```python
from build123d import *

# Parameters (mm, degrees)
F0_W     = 5.2
F0_H     = 226.71
F1_DEPTH = 2
F3_DEPTH = 4.5
F4_W     = 1.2
F4_H     = 2.1
F5_DEPTH = 25
F6_W     = 185.5
F6_H     = 227.71
F6_W_2   = 2.7
F7_DEPTH = 1
F8_W     = 2
F8_H     = 226.71
F9_DEPTH = 1
F10_SIZE = 1


with BuildPart() as f1:
    # F0 (on Top) → F1 (new body)
    with BuildSketch(Plane.XY):
        with Locations((2.6, 113.355)):
            Rectangle(F0_W, F0_H)
        with Locations((63.6, 113.355)):
            Rectangle(F0_W, F0_H)
        with Locations((124.6, 113.355)):
            Rectangle(F0_W, F0_H)
    extrude(amount=F1_DEPTH)

    # F2 (on face) → F3 (join)
    with BuildSketch(Plane.XY.offset(2)):
        Polygon((0, 226.71), (0, 0), (2, 0), (2, 224.71), (3.2, 224.71), (3.2, 0), (5.2, 0), (5.2, 226.71), align=None)
        Polygon((61, 226.71), (61, 0), (63, 0), (63, 224.71), (64.2, 224.71), (64.2, 0), (66.2, 0), (66.2, 226.71), align=None)
        Polygon((122, 226.71), (122, 0), (124, 0), (124, 224.71), (125.2, 224.71), (125.2, 0), (127.2, 0), (127.2, 226.71), align=None)
    extrude(amount=F3_DEPTH)

    # F4 (on face) → F5 (cut)
    with BuildSketch(Plane.XY.offset(2)):
        with Locations((2.6, 2.95)):
            Rectangle(F4_W, F4_H)
        with Locations((63.6, 2.95)):
            Rectangle(F4_W, F4_H)
        with Locations((124.6, 2.95)):
            Rectangle(F4_W, F4_H)
    extrude(amount=-F5_DEPTH, mode=Mode.SUBTRACT)

    # F6 (on Top) → F7 (join)
    with BuildSketch(Plane.XY):
        with Locations((34.45, 113.855)):
            Rectangle(F6_W, F6_H)
        with Locations((128.55, 113.855)):
            Rectangle(F6_W_2, F6_H)
    extrude(amount=-F7_DEPTH)

    # F8 (on face) → F9 (join)
    with BuildSketch(Plane.XY):
        with Locations((-53.8, 113.355)):
            Rectangle(F8_W, F8_H)
    extrude(amount=F9_DEPTH)

    # F10
    f10_edges = [f1.edges().sort_by_distance(p)[0] for p in [
        (2.6, 0, 2),
        (63.6, 0, 2),
        (124.6, 0, 2),
    ]]
    chamfer(f10_edges, length=F10_SIZE)


solid = f1.part
```
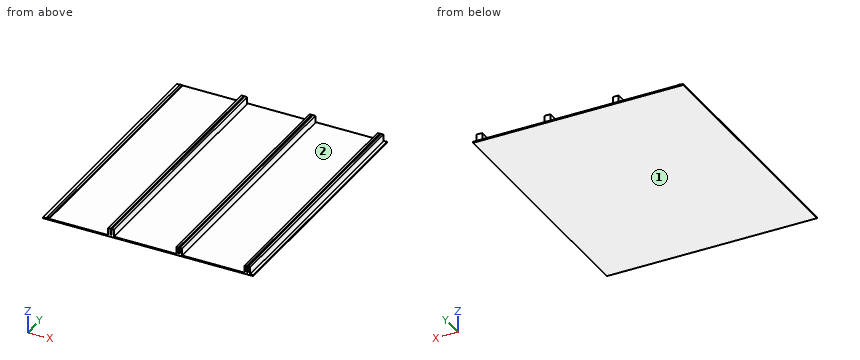
Here's how the part is built. I have some questions about the finished solid (model axes, mm). Face numbers are marked on the shaded views. Give positions to 0.01 mm unless a question says otherwise; leave off trailing zeros. Loops run counter-clockwise (first coordinate to the right, second up) from the corner with the lowest first, then second, coordinate; pieces in that order, holes last. Notation, with made-up numbers: M 67.25,67 L 114.25,67 A20 cw 114.25,102 Z; hole C -37,36 d2. An arc over 180 degrees is marked long. Put each result on its own line as item: value. Start each with the question number.
(1) I want a section at A-A on z = 4.25. Please give me the cut outline in (x, y).
(2) Will these pins go through, and if not, where does the flat tip stop? pin 1 Ø0.6 at (x, y) = (2.5, 133) entering from +Z; pin 2 Ø2 at (y, z) = (98, 1.5) entering from -X; pin 3 Ø2 at (y, z) = (98.5, 2) entering from +X; pin 4 Ø4 at (x, z) = (57.5, 3) entering from -Y.
(3) I want a section at C-C on x = 95. Please give me the cut outline in (y, z).
(4) If we mould it in two halves opening along X, with no side actions, what happens to the marked faces 1 and 2? For each: +X half, -X half, draft (parallel to the pull), parting line (faces both ways), or undercut.
(5) I need wall thicknesses on line 1 along X through (y, z) = (148, 3); line 2 along X through (y, z) = (114, 0.5); line 3 along X through (y, z) = (82, 1.5). Which ranges of each line are inside material? Lowest first, please. Write a range as [from, to].
Answer block:
1. outline: M 0,0 L 2,0 L 2,224.71 L 3.2,224.71 L 3.2,0 L 5.2,0 L 5.2,226.71 L 0,226.71 Z; M 61,0 L 63,0 L 63,224.71 L 64.2,224.71 L 64.2,0 L 66.2,0 L 66.2,226.71 L 61,226.71 Z; M 122,0 L 124,0 L 124,224.71 L 125.2,224.71 L 125.2,0 L 127.2,0 L 127.2,226.71 L 122,226.71 Z
2. pin 1: z = 2
2. pin 2: x = -54.8
2. pin 3: x = 127.2
2. pin 4: through
3. outline: M 0,-1 L 227.71,-1 L 227.71,0 L 0,0 Z
4. face 1: draft
4. face 2: undercut
5. line 1: [0, 2], [3.2, 5.2], [61, 63], [64.2, 66.2], [122, 124], [125.2, 127.2]
5. line 2: [-54.8, -52.8], [0, 5.2], [61, 66.2], [122, 127.2]
5. line 3: [0, 5.2], [61, 66.2], [122, 127.2]
